Could you check a few things on this drawing? It's one solid part, dimensions in mm from its lowest x, y, z. Give positions to 0.01 mm unless a question says otherwise; leave off trailing zeros. Write each loop counter-clockwise with the first axis right and the second up, starting at its lowest first coordinate (ties: lowest second). Pieces come first, ordered by that corner, then holes. Notation, with made-up numbers: (39, 85.25) -> (90, 85.25) arc R31 ccw to (90, 112.25) -> close; hole circle Ø1 at (78, 12). An arc over 180 degrees is marked (long way). Answer as CSV lines item,"result". Start each with the question number.
1. I'm going to push flat-ended pins straight in: P1, Ø2, axis at x = 39.5, y = 59.5, coming from the +Z side; P2, Ø2, axis at y = 35, z = 4.5, coming from the +X side; P3, Ø1.5, axis at y = 83, z = 1.5, coming from the -X side. Where does each tip first touch, or does it pass through?
2. If we section it at B-B on x = 51.21: Write out the boundary of the cut face in (y, z) (3 decimals), plus the area to 3 significant figures.
3. If we mould it in two halves opening along Y, with no side actions, what happens to the marked faces 1 and 2? For each: pulls with the +Y half, pulls with the -Y half, needs draft (parallel to the pull), parting line crosses it, or undercut.
4. If we section it at D-D on z = 2.25: Write out the boundary of the cut face in (x, y) (3 decimals), plus the area to 3 significant figures.
5. If we section it at A-A on x = 17.5: Write out the boundary of the cut face in (y, z) (3 decimals), plus the area to 3 significant figures.
6. I need wall thicknesses on line 1 (Y direction, x = 11.81, z = 0.8) (3 decimals); line 2 (Y direction, x = 47, z = 3.9) (3 decimals); line 3 (Y direction, x = 20.5, z = 2.3) (3 decimals). Which ranges of each line are inside material? Lowest first, please. Write a range as [from, to].
7. If we section it at C-C on y = 77: Write out the boundary of the cut face in (x, z), plus the area to 3 significant figures.
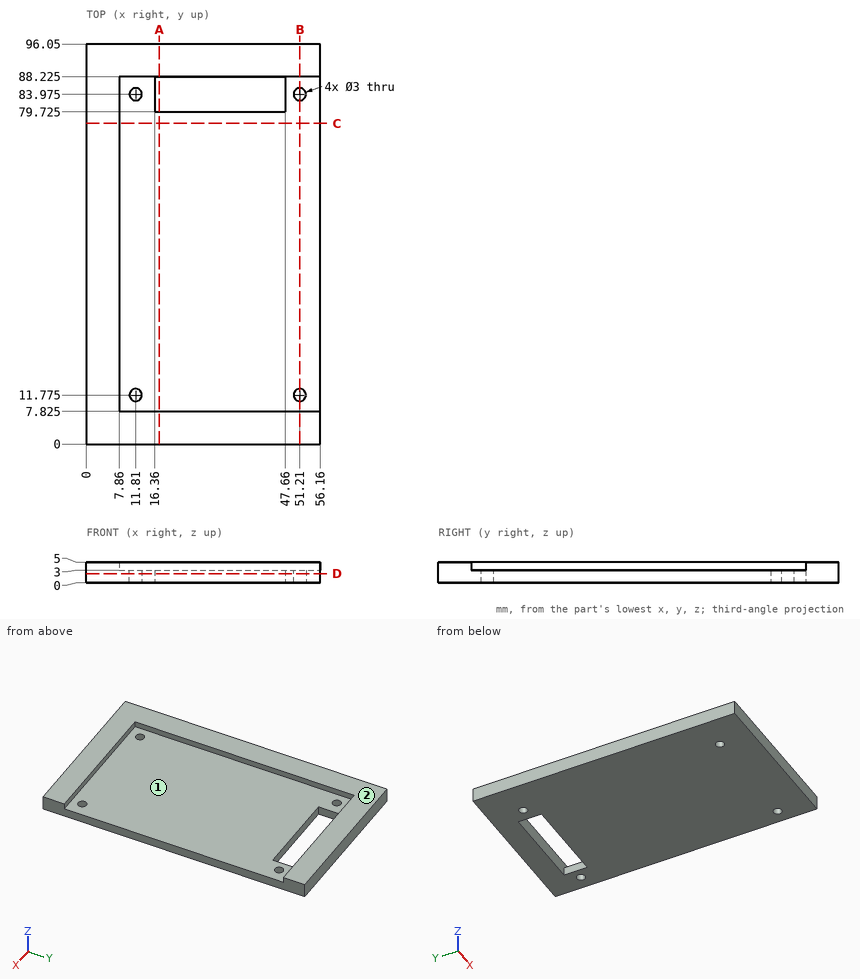
Computed values:
1,P1,"stops at z = 3"
1,P2,"stops at x = 7.86"
1,P3,"stops at x = 0"
2,outline,"(0, 0) -> (10.275, 0) -> (10.275, 3) -> (7.825, 3) -> (7.825, 5) -> (0, 5) -> close; (13.275, 0) -> (82.475, 0) -> (82.475, 3) -> (13.275, 3) -> close; (85.475, 0) -> (96.05, 0) -> (96.05, 5) -> (88.225, 5) -> (88.225, 3) -> (85.475, 3) -> close"
2,area,"301 mm2"
3,face 1,"undercut"
3,face 2,"needs draft"
4,outline,"(0, 0) -> (56.16, 0) -> (56.16, 96.05) -> (0, 96.05) -> close; hole circle Ø3 at (11.81, 11.775); hole circle Ø3 at (11.81, 83.975); hole (16.36, 79.725) -> (47.66, 79.725) -> (47.66, 88.225) -> (16.36, 88.225) -> close; hole circle Ø3 at (51.21, 11.775); hole circle Ø3 at (51.21, 83.975)"
4,area,"5,100 mm2"
5,outline,"(0, 0) -> (79.725, 0) -> (79.725, 3) -> (7.825, 3) -> (7.825, 5) -> (0, 5) -> close; (88.225, 0) -> (96.05, 0) -> (96.05, 5) -> (88.225, 5) -> close"
5,area,"294 mm2"
6,line 1,"y = [0, 10.275], [13.275, 82.475], [85.475, 96.05]"
6,line 2,"y = [0, 7.825], [88.225, 96.05]"
6,line 3,"y = [0, 79.725], [88.225, 96.05]"
7,outline,"(0, 0) -> (56.16, 0) -> (56.16, 3) -> (7.86, 3) -> (7.86, 5) -> (0, 5) -> close"
7,area,"184 mm2"
